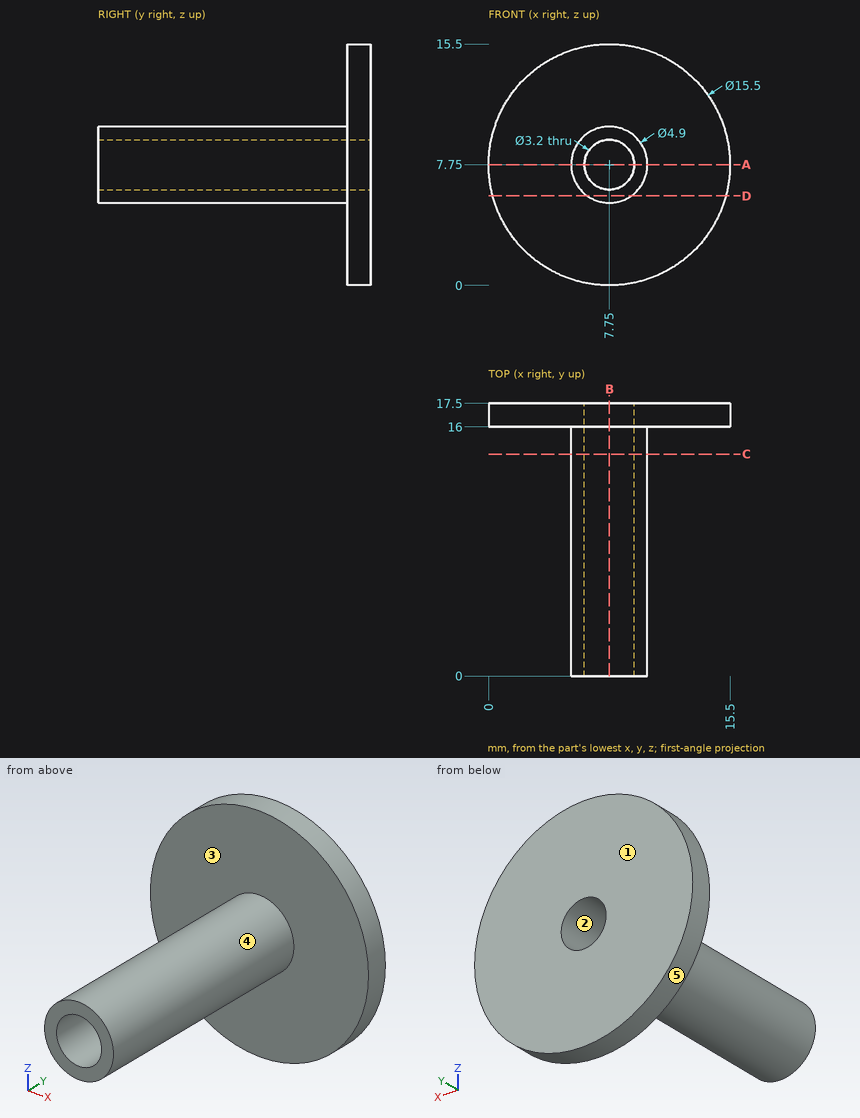
Geometry check sheet. Reference: drawing and pictorial views, mm from the part's lowest x, y, z. A direction names the side the tool comes from. Coordinates: 2 decimals unless noted, no trailing zeros. Write each loop counter-clockwise with the first axis right and the second up, starting at its lowest first coordinate (ties: lowest second). Pieces come first, ordered by that corner, then holes. Notation, with made-up numbers: (58, -18) -> (99, -18) arc R29 cw to (99, 10) -> close; hole circle Ø11 at (-10, -35). An arc over 180 degrees is marked (long way). One line per question, with ' | ' between items.
1. Cross-section at A-A on z = 7.75. Record the cut outline in (x, y), and give its area (4 significant figures).
Answers:
outline: (0, 16) -> (5.3, 16) -> (5.3, 0) -> (6.15, 0) -> (6.15, 17.5) -> (0, 17.5) -> close; (9.35, 0) -> (10.2, 0) -> (10.2, 16) -> (15.5, 16) -> (15.5, 17.5) -> (9.35, 17.5) -> close | area: 45.65 mm²
2. Draft check along Y on the marked faces 1, 2 and 3. Enter one of: +Y half, -Y half, draft (parallel to the pull), parting line (faces both ways), or undercut.
Answers:
face 1: +Y half | face 2: draft | face 3: -Y half
3. Cross-section at B-B on x = 7.75. Record the cut outline in (y, z).
Answers:
outline: (0, 5.3) -> (16, 5.3) -> (16, 0) -> (17.5, 0) -> (17.5, 6.15) -> (0, 6.15) -> close; (0, 9.35) -> (17.5, 9.35) -> (17.5, 15.5) -> (16, 15.5) -> (16, 10.2) -> (0, 10.2) -> close
4. Depth check by flat-ended pin: pin 1 Ø6 at (x, y) = (3.5, 5) entering from -Z; pin 2 Ø8 at (x, y) = (5, 3.5) entering from -Z; pin 3 Ø3 at (y, z) = (12.5, 10) entering from -X; pin 4 Ø3 at (x, z) = (7.75, 7.75) entering from -Y. Enter the tip coordinate at first touch or a pass-through.
Answers:
pin 1: stops at z = 5.64 | pin 2: stops at z = 5.3 | pin 3: stops at x = 5.42 | pin 4: passes through
5. Cross-section at D-D on z = 5.75. Record the cut outline in (x, y).
Answers:
outline: (0.26, 16) -> (6.33, 16) -> (6.33, 0) -> (9.17, 0) -> (9.17, 16) -> (15.24, 16) -> (15.24, 17.5) -> (0.26, 17.5) -> close
6. Thickness scan on probe 1 along X at (y, z) = (9.5, 7.75); probe 2 along Y at (x, z) = (3.25, 7.5); probe 3 along X at (y, z) = (6.75, 9). Record the ranges inside material, lowest first. Write a range as from..to.
Answers:
probe 1: x = 5.3..6.15, 9.35..10.2 | probe 2: y = 16..17.5 | probe 3: x = 5.64..6.75, 8.75..9.86
7. Cross-section at C-C on y = 14.25. Record the cut outline in (x, z), and give its area (3 significant figures).
Answers:
outline: circle Ø4.9 at (7.75, 7.75); hole circle Ø3.2 at (7.75, 7.75) | area: 10.8 mm²
8. Set-up check for the marked faces 4 and 5: record each of +Z, -Z, +X, -X, +Y, -Y from which the full face is reachable in a straight line by a thin tool's end or side.
Answers:
face 4: -Y | face 5: +Y, -Y
